Could you check a few things on this drawing? It's one solid part, dimensions in mm from its lowest x, y, z. A direction names the side the tool comes from. Give positions to 0.01 mm unless a question says otherwise; leave off trailing zeros. Order: outer loops, then holes, each group sorted by start corner. A loop starts at its lowest first (then second) coordinate and runs counter-clockwise, first axis right, second up. Notation, with made-up numbers: (-34, 43.25) -> (-29, 43.25) arc R10 cw to (-29, 58.25) -> close; hole circle Ø3 at (53, 38.25). An arc over 180 degrees is marked (long way). Write each question's results on one line, items separated by ' | '. Start each with the question number.
Q1. Imagine slicing it at A-A, the plane x = 12.7. Please give me the cut outline in (y, z) (1 decimal), then the cut area to 3 significant figures.
Q2. For the marked faces 1 and 2, which set-ups out of +Z, -Z, +X, -X, +Y, -Y let a thin tool reach every point of the face, with its end or its side?
Q3. Imagine slicing it at C-C, the plane z = 38.1. Please give me the cut outline in (x, y) (3 decimals), then the cut area to 3 significant figures.
Q4. I need wall thicknesses on line 1 along X through (y, z) = (23.55, 38.1) (3 decimals); line 2 along Y through (x, z) = (23, 20) (3 decimals); line 3 along X through (y, z) = (1.1, 12.7) (3 decimals). Which ranges of each line are inside material? Lowest first, please. Write a range as [from, to].
Q5. Imagine slicing it at B-B, the plane x = 114.3. Please give me the cut outline in (y, z) (3 decimals), then the cut area to 3 significant figures.
Q6. Imagine slicing it at D-D, the plane z = 25.4. Please give me the cut outline in (x, y) (1 decimal), then the cut area to 3 significant figures.
Q7. I'm going to push flat-ended pins straight in: pin 1 (3.5 mm diameter, centred on y = 10, z = 49.5, fed in from +X); pin 2 (1.5 mm diameter, centred on y = 16, z = 6.5, fed in from +X) (3 decimals). Where does each tip first touch, or does it pass through?
Q8. Thinking about a two-plate mould opening in Y: for the marked faces 3, 4, 5 and 6, which applies, pulls with the +Y half, pulls with the -Y half, needs draft (parallel to the pull), parting line crosses it, or undercut?
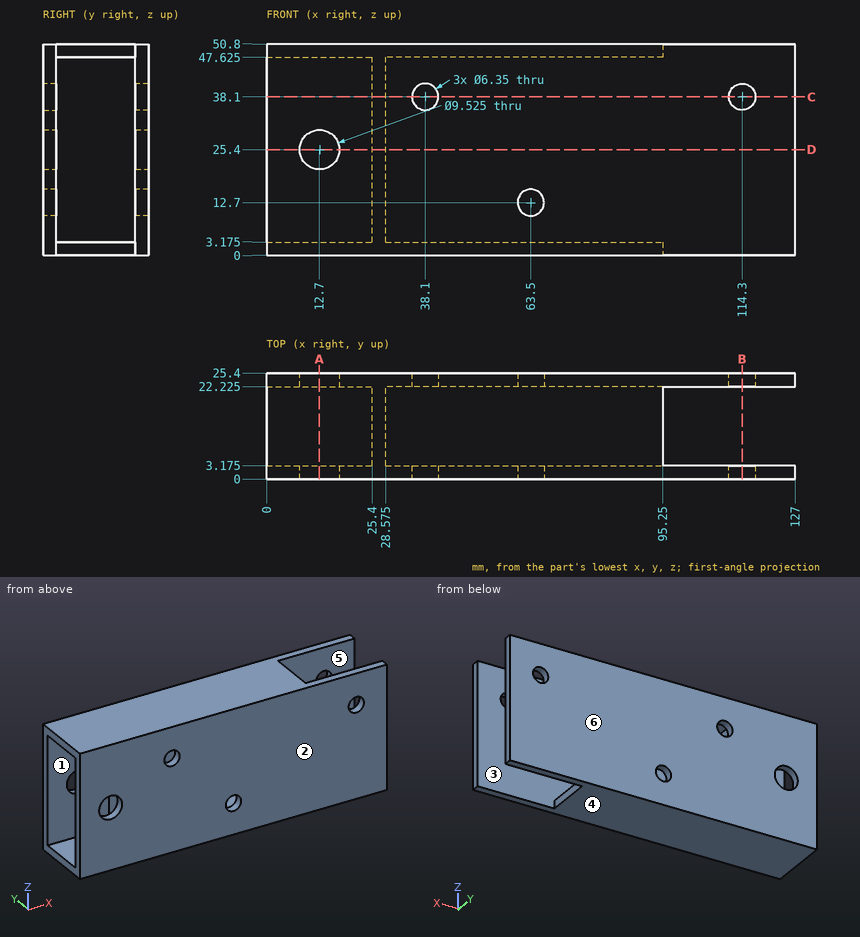
Geometry check:
1) outline: (0, 0) -> (25.4, 0) -> (25.4, 20.6) -> (22.2, 20.6) -> (22.2, 3.2) -> (3.2, 3.2) -> (3.2, 20.6) -> (0, 20.6) -> close; (0, 30.2) -> (3.2, 30.2) -> (3.2, 47.6) -> (22.2, 47.6) -> (22.2, 30.2) -> (25.4, 30.2) -> (25.4, 50.8) -> (0, 50.8) -> close | area: 383 mm²
2) face 1: -X | face 2: +Z, -Z, +X, -X, -Y
3) outline: (0, 0) -> (34.925, 0) -> (34.925, 3.175) -> (28.575, 3.175) -> (28.575, 22.225) -> (34.925, 22.225) -> (34.925, 25.4) -> (0, 25.4) -> (0, 22.225) -> (25.4, 22.225) -> (25.4, 3.175) -> (0, 3.175) -> close; (41.275, 0) -> (111.125, 0) -> (111.125, 3.175) -> (41.275, 3.175) -> close; (41.275, 22.225) -> (111.125, 22.225) -> (111.125, 25.4) -> (41.275, 25.4) -> close; (117.475, 0) -> (127, 0) -> (127, 3.175) -> (117.475, 3.175) -> close; (117.475, 22.225) -> (127, 22.225) -> (127, 25.4) -> (117.475, 25.4) -> close | area: 786 mm²
4) line 1: [0, 34.925], [41.275, 111.125], [117.475, 127] | line 2: [0, 3.175], [22.225, 25.4] | line 3: [0, 60.325], [66.675, 127]
5) outline: (0, 0) -> (3.175, 0) -> (3.175, 34.925) -> (0, 34.925) -> close; (0, 41.275) -> (3.175, 41.275) -> (3.175, 50.8) -> (0, 50.8) -> close; (22.225, 0) -> (25.4, 0) -> (25.4, 34.925) -> (22.225, 34.925) -> close; (22.225, 41.275) -> (25.4, 41.275) -> (25.4, 50.8) -> (22.225, 50.8) -> close | area: 282 mm²
6) outline: (0, 0) -> (7.9, 0) -> (7.9, 3.2) -> (0, 3.2) -> close; (0, 22.2) -> (7.9, 22.2) -> (7.9, 25.4) -> (0, 25.4) -> close; (17.5, 0) -> (127, 0) -> (127, 3.2) -> (28.6, 3.2) -> (28.6, 22.2) -> (127, 22.2) -> (127, 25.4) -> (17.5, 25.4) -> (17.5, 22.2) -> (25.4, 22.2) -> (25.4, 3.2) -> (17.5, 3.2) -> close | area: 806 mm²
7) pin 1: x = 95.25 | pin 2: x = 28.575
8) face 3: undercut | face 4: needs draft | face 5: undercut | face 6: pulls with the +Y half
